Autodesk Inventor part; units mm, degrees
ref_plane "YZ Plane" through (0, 0, 0) normal (1, 0, 0) x (0, 1, 0)
ref_plane "XZ Plane" through (0, 0, 0) normal (0, 1, 0) x (-1, 0, 0)
ref_plane "XY Plane" through (0, 0, 0) normal (0, 0, 1) x (1, 0, 0)
sketch "Sketch1" plane through (0, 0, 0) normal (0, 0, 1) x (1, 0, 0)
  line L0 (0, 0) -> (190.5, 0) construction
  line L1 (190.5, 0) -> (190.5, 152.4) construction
  line L2 (190.5, 152.4) -> (0, 152.4) construction
  line L3 (0, 152.4) -> (0, 0) construction
  line L4 (0, 0) -> (190.5, 0)
  line L5 (0, 0) -> (0, 38.1)
  line L6 (0, 0) -> (38.1, 0) construction
  line L7 (190.5, 0) -> (190.5, 38.1)
  line L8 (190.5, 0) -> (228.6, 0) construction
  line L9 (190.5, 152.4) -> (38.1, 152.4) construction
  line L10 (190.5, 152.4) -> (342.9, 152.4) construction
  line L11 (38.1, 152.4) -> (0, 152.4) construction
  line L12 (0, 38.1) -> (0, 152.4)
  line L13 (0, 152.4) -> (38.1, 152.4)
  line L14 (38.1, 152.4) -> (190.5, 38.1)
  circle A0 centre (12.7, 25.4) radius 3.175
  circle A1 centre (63.5, 25.4) radius 3.175
  circle A2 centre (12.7, 139.7) radius 3.175
  circle A3 centre (25.4, 127) radius 3.175
  circle A4 centre (12.7, 114.3) radius 3.175
  circle A5 centre (25.4, 101.6) radius 3.175
  circle A6 centre (114.3, 25.4) radius 3.175
  circle A7 centre (165.1, 25.4) radius 3.175
  dimension "d0" = 190.5
  dimension "d1" = 152.4
  dimension "d2" = 12.7
  dimension "d3" = 50.8
  dimension "d8" = 25.4
  dimension "d9" = 25.4
  dimension "d10" = 38.1
  dimension "d11" = 90
  dimension "d12" = 38.1
  dimension "d13" = 90
  dimension "d14" = 152.4
  dimension "d15" = 180
  dimension "d16" = 38.1
  dimension "d17" = 12.7
  dimension "d18" = 12.7
  dimension "d19" = 12.7
  dimension "d20" = 12.7
  dimension "d21" = 12.7
  dimension "d22" = 25.4
  dimension "d23" = 38.1
  dimension "d24" = 50.8
  dimension "d25" = 6.35
  dimension "d26" = 6.35
  dimension "d29" = 6.35
  dimension "d30" = 6.35
  dimension "d31" = 6.35
  dimension "d32" = 6.35
  dimension "d35" = 50.8
  dimension "d36" = 50.8
  dimension "d38" = 6.35
  dimension "d39" = 6.35
  dimension "d46" = 25.4
  dimension "d47" = 25.4
extrude "Extrusion4" add sketch "Sketch1" along normal blind 6.35
sketch "Sketch3" plane through (0, 0, 6.35) normal (0, 0, 1) x (1, 0, 0)
  line L0 (0, 0) -> (0, 25.4)
  line L1 (0, 152.4) -> (0, 0)
  line L2 (0, 0) -> (12.7, 0)
  line L3 (0, 0) -> (190.5, 0)
  line L4 (0, 25.4) -> (12.7, 0)
  point P0 (0, 38.1)
  dimension "d50" = 25.4
  dimension "d51" = 12.7
extrude "Extrusion5" cut sketch "Sketch3" against normal blind 6.35
sketch "Sketch4" plane through (0, 0, 6.35) normal (0, 0, 1) x (1, 0, 0)
  line L0 (0, 152.4) -> (0, 25.4)
  line L1 (12.7, 0) -> (190.5, 0)
  circle A0 centre (9.525, 52.3875) radius 3.175
  circle A1 centre (25.4, 52.3875) radius 3.175
  circle A2 centre (19.05, 69.85) radius 4.7625
  point P0 (0, 0)
  point P1 (0, 38.1)
  dimension "d54" = 9.525
  dimension "d55" = 25.4
  dimension "d56" = 52.3875
  dimension "d57" = 52.3875
  dimension "d58" = 69.85
  dimension "d59" = 19.05
  dimension "d60" = 6.35
  dimension "d61" = 6.35
  dimension "d62" = 9.525
extrude "Extrusion6" cut sketch "Sketch4" against normal blind 6.35
properties part number "rail mounting bracket"
Input: part model. Units: mm. Frame: model coordinates. Round coordinates to 2 decimals unless told otherwise and drop trailing zeros. Loops run counter-clockwise (first coordinate to the right, second up) from the corner with the lowest first, then second, coordinate; pieces in that order, holes last. Notation, with made-up numbers: (17, -34.5) -> (45, -34.5) arc R10 ccw to (45, -17.5) -> close; hole circle Ø1 at (30.5, 46). An arc over 180 degrees is marked (long way). Answer as a JSON object with one key per item and string values. Group by question number.
1) Section query A-A on x = 165.1. Output: boundary loops of the cut face in (y, z) (3 decimals).
2) Ray query, L1, parallel to Y at x = 25.4, z = 2 (1 decimal); L2, parallel to Y at x = 26, z = 3.5; L3, parallel to X at y = 139.7, z = 5 (3 decimals). Return the intervals inside material, ascending.
3) Pin query (flat end, axial travel): pin 1 (3 mm diameter, centred on y = 89, z = 3, fed in from +X); pin 2 (2 mm diameter, centred on y = 58, z = 1, fed in from +X). Return the tip coordinate at first contact, or that it passes through.
4) Section query B-B on y = 114.3. Output: boundary loops of the cut face in (x, z) (3 decimals), plus the area to 3 significant figures.
5) Section query D-D on x = 107.5. Output: boundary loops of the cut face in (y, z).
6) Section query C-C on z = 2.25. State how many separate pieces and enclosed holes the cut face has, plus the area to 3 significant figures.
7) Draft query along Y for faces 1 (the flat face through (100, 0, 3)), 2 (the flat face through (73, 60, 0)), 3 (the cylindrical face through (117.33, 24.45, 3.13)). Return one class per face: +Y half, -Y half, draft (parallel to the pull), parting line (faces both ways), or undercut.
Reply:
{
 "1": {"outline": "(0, 0) -> (22.225, 0) -> (22.225, 6.35) -> (0, 6.35) -> close; (28.575, 0) -> (57.15, 0) -> (57.15, 6.35) -> (28.575, 6.35) -> close"},
 "2": {"L1": "y = 0 to 49.2, 55.6 to 98.4, 104.8 to 123.8, 130.2 to 152.4", "L2": "y = 0 to 49.27, 55.51 to 98.48, 104.72 to 123.88, 130.12 to 152.4", "L3": "x = 0 to 9.525, 15.875 to 55.033"},
 "3": {"pin 1": "stops at x = 124.63", "pin 2": "stops at x = 165.3"},
 "4": {"outline": "(0, 0) -> (9.525, 0) -> (9.525, 6.35) -> (0, 6.35) -> close; (15.875, 0) -> (88.9, 0) -> (88.9, 6.35) -> (15.875, 6.35) -> close", "area": "524 mm2"},
 "5": {"outline": "(0, 0) -> (100.35, 0) -> (100.35, 6.35) -> (0, 6.35) -> close"},
 "6": {"separate pieces": "1", "enclosed holes": "11", "area": "19,800 mm2"},
 "7": {"face 1": "-Y half", "face 2": "draft", "face 3": "undercut"}
}
